Part print with two shaded views. Sizes in mm from the minimum x, y, z corner. A direction names the side the tool comes from. Coordinates: 2 decimals unless noted, no trailing zeros. Loops run counter-clockwise (first coordinate to the right, second up) from the corner with the lowest first, then second, coordinate; pieces in that order, holes last.
(1) Slice it at A-A (z = 32). Give the cut face in (x, y) (1 decimal).
(2) Two-plate mould, pull along Z, no slides. Class the marked faces 5, 6 and 7: pulls with the +Z half, pulls with the -Z half, needs draft (parallel to the pull), parting line crosses it, or undercut.
(3) Slice it at B-B (y = 5.5). Give the cut face in (x, z) (1 decimal).
(4) Wall check: L1, parallel to Z at x = 17.5, y = 4 (1 decimal); L2, parallel to Z at x = 25.5, y = 23.5 (1 decimal); L3, parallel to Y at x = 19.5, z = 24.5 (1 decimal). Give the ranges that are in metal, low to high.
(5) Flat gauge pins, fed straight in: P1, Ø5, axis at y = 17.5, z = 22.5, coming from the -X side; P2, Ø5.5, axis at x = 17, z = 20.5, coming from the -Y side (1 decimal); P3, Ø7.5, axis at x = 14.5, z = 35.5, coming from the +Y side; P4, Ø2, axis at y = 30.5, z = 37, coming from the -X side. Where does each tip first touch, or does it go through?
(6) Tool access for the marked faces 1, 2, 3 and 4: list every direction of +Z, -Z, +X, -X, +Y, -Y with a clear straight run to the whole face (end or side of a thin tool).
(7) Slice it at C-C (z = 16). Give the cut face in (x, y) (1 decimal).
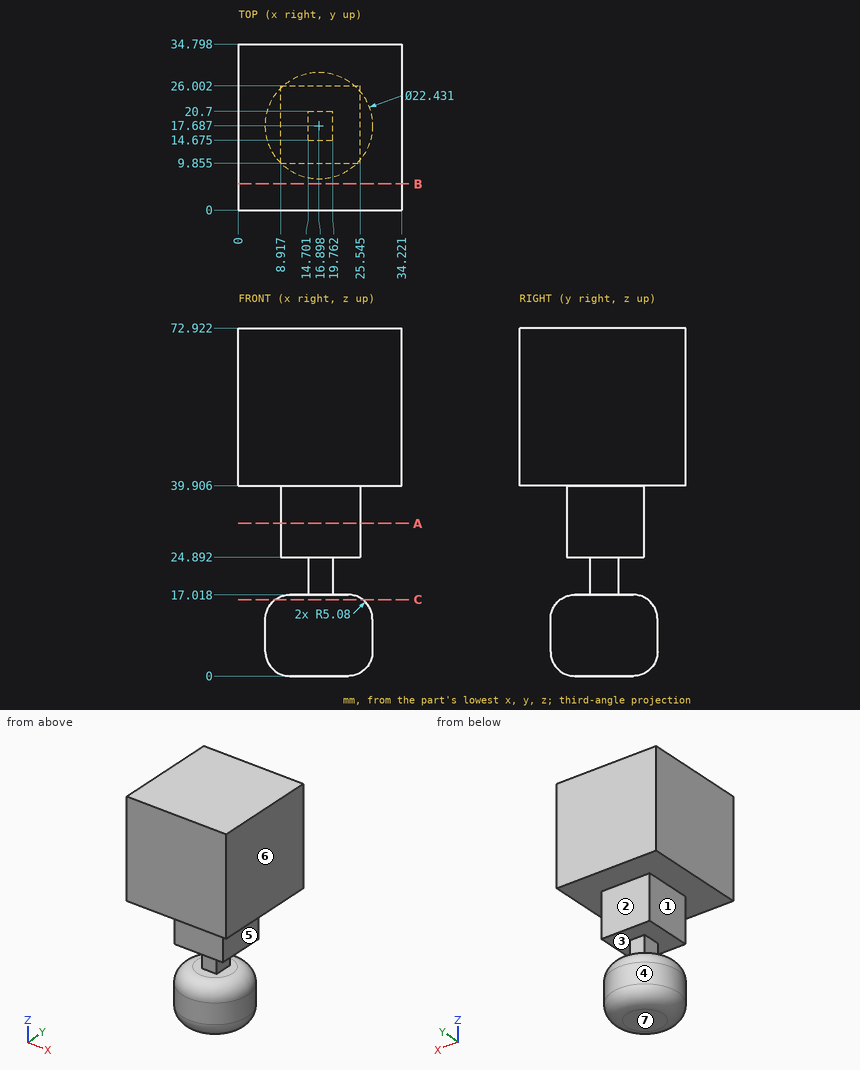
Response values:
1. outline: (8.9, 9.9) - (25.5, 9.9) - (25.5, 26) - (8.9, 26) - close
2. face 5: undercut
2. face 6: needs draft
2. face 7: pulls with the -Z half
3. outline: (0, 39.9) - (34.2, 39.9) - (34.2, 72.9) - (0, 72.9) - close
4. L1: z = 39.9 to 72.9
4. L2: z = 2.3 to 14.7, 24.9 to 72.9
4. L3: y = 14.7 to 20.7
5. P1: stops at x = 8.92
5. P2: stops at y = 14.7
5. P3: stops at y = 26
5. P4: passes through
6. face 1: -X, +Y, -Y
6. face 2: +X, -X, +Y
6. face 3: none
6. face 4: -Z
7. outline: circle Ø18.4 at (16.9, 17.7)
